Here's the drawing with two shaded views (mm, measured from the low corner). I have some questions. Coordinates: 2 decimals unless noted, no trailing zeros. Write each loop counter-clockwise with the first axis right and the second up, starting at its lowest first coordinate (ties: lowest second). Pieces come first, ordered by that corner, then holes.
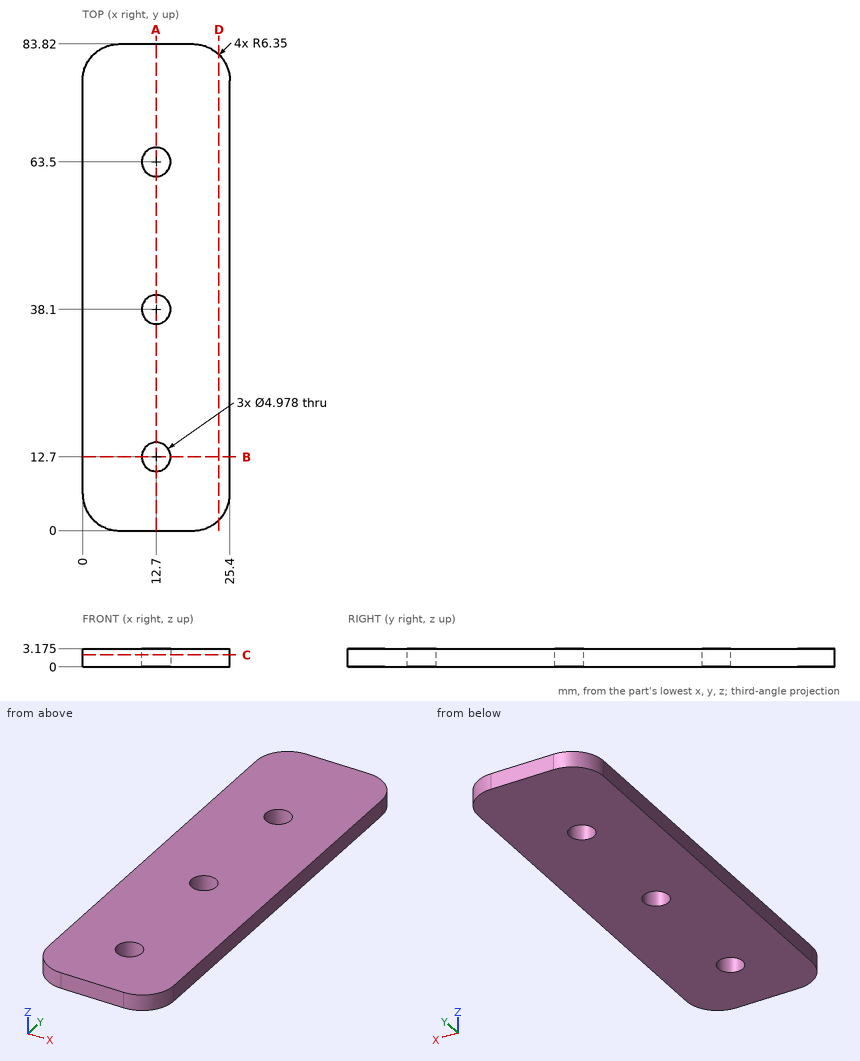
1. Please list where these lines run through material, in increasing order: line 1 along Y through (x, z) = (12.7, 1.9); line 2 along X through (y, z) = (38, 0.9); line 3 along Y through (x, z) = (14.5, 2.9).
Verdict:
line 1: y = 0 to 10.21, 15.19 to 35.61, 40.59 to 61.01, 65.99 to 83.82
line 2: x = 0 to 10.21, 15.19 to 25.4
line 3: y = 0 to 10.98, 14.42 to 36.38, 39.82 to 61.78, 65.22 to 83.82
2. I want a section at A-A on x = 12.7. Please give me the cut outline in (y, z) (1 decimal).
Verdict:
outline: (0, 0) - (10.2, 0) - (10.2, 3.2) - (0, 3.2) - close; (15.2, 0) - (35.6, 0) - (35.6, 3.2) - (15.2, 3.2) - close; (40.6, 0) - (61, 0) - (61, 3.2) - (40.6, 3.2) - close; (66, 0) - (83.8, 0) - (83.8, 3.2) - (66, 3.2) - close
3. I want a section at D-D on x = 23.5. Please give me the cut outline in (y, z) (1 decimal).
Verdict:
outline: (1.8, 0) - (82, 0) - (82, 3.2) - (1.8, 3.2) - close
4. I want a section at C-C on z = 2.1. Please give me the cut outline in (x, y), plus the area to 3 significant figures.
Verdict:
outline: (0, 6.35) arc R6.35 ccw to (6.35, 0) - (19.05, 0) arc R6.35 ccw to (25.4, 6.35) - (25.4, 77.47) arc R6.35 ccw to (19.05, 83.82) - (6.35, 83.82) arc R6.35 ccw to (0, 77.47) - close; hole circle Ø4.98 at (12.7, 12.7); hole circle Ø4.98 at (12.7, 38.1); hole circle Ø4.98 at (12.7, 63.5)
area: 2,040 mm2
5. I want a section at B-B on y = 12.7. Please give me the cut outline in (x, z) (1 decimal).
Verdict:
outline: (0, 0) - (10.2, 0) - (10.2, 3.2) - (0, 3.2) - close; (15.2, 0) - (25.4, 0) - (25.4, 3.2) - (15.2, 3.2) - close
